Geometry check sheet. Reference: the model listing, model coordinates, mm. Face numbers are marked on the shaded views. A direction names the side the tool comes from. Round coordinates to 2 decimals unless told otherwise and drop trailing zeros. Loops run counter-clockwise (first coordinate to the right, second up) from the corner with the lowest first, then second, coordinate; pieces in that order, holes last. Notation, with made-up numbers: (-21.5, 23.5) - (25.5, 23.5) arc R20 ccw to (25.5, 59.5) - close; hole circle Ø3 at (-2.75, 50). An arc over 180 degrees is marked (long way). Answer as CSV lines item,"result". Start each with the question number.
1) Draft check along X on the marked faces 5, 6 and 7. Enter one of: released by +X, released by -X, zero draft, split by the parting line, or undercut.
2) Depth check by flat-ended pin: P1, Ø3.5, axis at x = -10.5, z = 36.5, coming from the -Y side; P2, Ø1.6, axis at x = 3.5, z = 26, coming from the -Y side; P3, Ø3, axis at x = -7.5, z = 26.5, coming from the -Y side. Enter the tip coordinate at first touch or a pass-through.
3) Cross-section at B-B on x = -0.5. Record the boundary of the cut face in (y, z), and give its area (3 significant figures).
4) Cross-section at D-D on x = 5. Record the boundary of the cut face in (y, z), and give its area (3 significant figures).
5) Cross-section at C-C on z = 32.75. Record the boundary of the cut face in (x, y).
6) Access from +Z, -Z, +X, -X, +Y, -Y to the whole of each face (thin tool, end or side, straight path). Record for the marked faces 1, 2, 3 and 4.
7) Cross-section at A-A on y = -4.5. Record the boundary of the cut face in (x, z).
8) Thickness scan on line 1 along Y through (x, z) = (-3.5, 31); line 2 along X through (y, z) = (-2, 27.25); line 3 along X through (y, z) = (-10.25, 30.75). Record the ranges inside material, lowest first.
from build123d import *

# Parameters (mm, degrees)
F0_DEPTH = 3
F5_DEPTH = 9
F1_W     = 7
F1_H     = 2
F6_DEPTH = 3
F2_R     = 2.75
F2_R_2   = 1.5
F3_DEPTH = 1.5


with BuildPart() as f0:
    # F4 (on Front) → F0 (new body)
    with BuildSketch(Plane.XZ):
        with BuildLine():
            ThreePointArc((-5.3789273798, 23.6677408814), (-6.4395875516, 26.2284010532), (-3.8789273798, 25.1677408814))
            Line((-3.8789273798, 25.1677408814), (1.1210726202, 25.1677408814))
            ThreePointArc((1.1210726202, 25.1677408814), (2.6210726202, 26.6677408814), (4.1210726202, 25.1677408814))
            ThreePointArc((4.1210726202, 25.1677408814), (3.6817327919, 24.1070807097), (2.6210726202, 23.6677408814))
            Line((2.6210726202, 23.6677408814), (2.6210726202, 21.1677408814))
            ThreePointArc((2.6210726202, 21.1677408814), (3.6817327919, 20.7284010532), (4.1210726202, 19.6677408814))
            Line((4.1210726202, 19.6677408814), (9.1210726202, 19.6677408814))
            Line((9.1210726202, 19.6677408814), (9.1210726202, 30.6677408814))
            Line((9.1210726202, 30.6677408814), (-11.8789273798, 30.6677408814))
            Line((-11.8789273798, 30.6677408814), (-11.8789273798, 19.6677408814))
            Line((-11.8789273798, 19.6677408814), (-6.8789273798, 19.6677408814))
            ThreePointArc((-6.8789273798, 19.6677408814), (-6.4395875516, 20.7284010532), (-5.3789273798, 21.1677408814))
            Line((-5.3789273798, 21.1677408814), (-5.3789273798, 23.6677408814))
        make_face()
        with BuildLine():
            Line((1.1210726202, 25.1677408814), (-3.8789273798, 25.1677408814))
            ThreePointArc((-3.8789273798, 25.1677408814), (-4.3182672081, 24.1070807097), (-5.3789273798, 23.6677408814))
            Line((-5.3789273798, 23.6677408814), (-5.3789273798, 21.1677408814))
            ThreePointArc((-5.3789273798, 21.1677408814), (-4.3182672081, 20.7284010532), (-3.8789273798, 19.6677408814))
            Line((-3.8789273798, 19.6677408814), (1.1210726202, 19.6677408814))
            ThreePointArc((1.1210726202, 19.6677408814), (1.5604124484, 20.7284010532), (2.6210726202, 21.1677408814))
            Line((2.6210726202, 21.1677408814), (2.6210726202, 23.6677408814))
            ThreePointArc((2.6210726202, 23.6677408814), (1.5604124484, 24.1070807097), (1.1210726202, 25.1677408814))
        make_face()
    extrude(amount=F0_DEPTH)

    # F1 (on face) → F5 (join)
    with BuildSketch(Plane.XY.offset(30.6677408814)):
        Polygon((9.1210726202, 0), (-11.8789273798, 0), (-11.8789273798, -3), (-8.8789273798, -3), (-6.8789273798, -3), (4.1210726202, -3), (6.1210726202, -3), (9.1210726202, -3), align=None)
        Polygon((-8.8789273798, -3), (-11.8789273798, -3), (-11.8789273798, -12), (-8.8789273798, -12), (-8.8789273798, -11.5), (-8.8789273798, -9.5), (-8.8789273798, -5), align=None)
        Polygon((9.1210726202, -12), (9.1210726202, -3), (6.1210726202, -3), (6.1210726202, -5), (6.1210726202, -9.5), (6.1210726202, -11.5), (6.1210726202, -12), align=None)
    extrude(amount=F5_DEPTH)

    # F1 (on face) → F6 (join)
    with BuildSketch(Plane.XY.offset(30.6677408814)):
        Polygon((-8.8789273798, -11.5), (-8.8789273798, -12), (4.6210726202, -12), (6.1210726202, -12), (6.1210726202, -11.5), (4.1210726202, -11.5), (4.1210726202, -9.5), (6.1210726202, -9.5), (6.1210726202, -5), (4.1210726202, -5), (4.1210726202, -3), (-6.8789273798, -3), (-6.8789273798, -5), (-8.8789273798, -5), (-8.8789273798, -9.5), (-6.8789273798, -9.5), (-6.8789273798, -11.5), align=None)
        with Locations((-1.3789273798, -7.5)):
            Rectangle(F1_W, F1_H, mode=Mode.SUBTRACT)
        Polygon((-8.8789273798, -12), (-11.8789273798, -12), (-11.8789273798, -13.5), (9.1210726202, -13.5), (9.1210726202, -12), (6.1210726202, -12), (4.6210726202, -12), align=None)
    extrude(amount=F6_DEPTH)

    # F2 (on face) → F3 (cut)
    with BuildSketch(Plane.XZ.offset(3)):
        with Locations((2.6210726202, 25.1677408814)):
            Circle(F2_R)
        with Locations((2.6210726202, 25.1677408814)):
            Circle(F2_R_2, mode=Mode.SUBTRACT)
        with Locations((-5.3789273798, 25.1677408814)):
            Circle(F2_R)
        with Locations((-5.3789273798, 25.1677408814)):
            Circle(F2_R_2, mode=Mode.SUBTRACT)
    extrude(amount=-F3_DEPTH, mode=Mode.SUBTRACT)


solid = f0.part
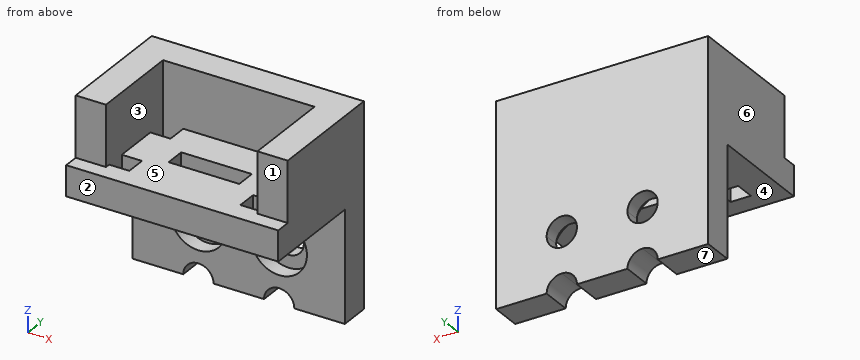
Answer block:
1,face 5,"undercut"
1,face 6,"released by -X"
1,face 7,"zero draft"
2,P1,"stops at y = -12"
2,P2,"stops at y = -1.5"
2,P3,"stops at y = -3"
3,outline,"(-13.5, 30.67) - (-8.5, 30.67) - (-8.5, 33.67) - (-13.5, 33.67) - close; (-6.5, 30.67) - (-3, 30.67) - (-3, 19.67) - (0, 19.67) - (0, 39.67) - (-3, 39.67) - (-3, 33.67) - (-6.5, 33.67) - close"
3,area,"85.5 mm^2"
4,outline,"(-13.5, 30.67) - (-11.5, 30.67) - (-11.5, 33.67) - (-13.5, 33.67) - close; (-9.5, 30.67) - (-5, 30.67) - (-5, 33.67) - (-9.5, 33.67) - close; (-3, 19.67) - (0, 19.67) - (0, 39.67) - (-3, 39.67) - (-3, 26.55) - (-1.5, 26.55) - (-1.5, 23.79) - (-3, 23.79) - close"
4,area,"75.4 mm^2"
5,outline,"(-11.88, -13.5) - (9.12, -13.5) - (9.12, 0) - (-11.88, 0) - close; hole (-8.88, -11.5) - (-6.88, -11.5) - (-6.88, -9.5) - (-8.88, -9.5) - close; hole (-8.88, -5) - (-6.88, -5) - (-6.88, -3) - (-8.88, -3) - close; hole (-4.88, -8.5) - (2.12, -8.5) - (2.12, -6.5) - (-4.88, -6.5) - close; hole (4.12, -11.5) - (6.12, -11.5) - (6.12, -9.5) - (4.12, -9.5) - close; hole (4.12, -5) - (6.12, -5) - (6.12, -3) - (4.12, -3) - close"
6,face 1,"+Z, +X, -X, -Y"
6,face 2,"+Z, -Z, +X, -X, -Y"
6,face 3,"+Z"
6,face 4,"-Z, +X, -X, -Y"
7,outline,"(-11.88, 30.67) - (-8.88, 30.67) - (-8.88, 39.67) - (-11.88, 39.67) - close; (-6.88, 30.67) - (4.12, 30.67) - (4.12, 33.67) - (-6.88, 33.67) - close; (6.12, 30.67) - (9.12, 30.67) - (9.12, 39.67) - (6.12, 39.67) - close"
8,line 1,"y = -13.5 to -8.5, -6.5 to 0"
8,line 2,"x = -11.88 to -7.18, -3.58 to 0.82, 4.42 to 9.12"
8,line 3,"x = -11.88 to -8.88, -6.88 to 4.12, 6.12 to 9.12"
